from build123d import *

# Parameters (mm, degrees)
SKETCH1_W                      = 86
SKETCH1_H                      = 16
BOSS_EXTRUDE1_DEPTH            = 3
M3_CLEARANCE_HOLE1_D           = 3.4
M3_CLEARANCE_HOLE1_CSINK_D     = 3.45
M3_CLEARANCE_HOLE1_CSINK_ANGLE = 90


with BuildPart() as part:
    # Sketch1 → Boss-Extrude1 (new body)
    with BuildSketch(Plane.XY):
        with Locations((43, 8)):
            Rectangle(SKETCH1_W, SKETCH1_H)
    extrude(amount=BOSS_EXTRUDE1_DEPTH)

    # M3 Clearance Hole1 (through all)
    with Locations(Plane.XY.offset(3)):
        with Locations((5.115834522, 13), (5.115834522, 3), (79.115834522, 13), (79.115834522, 3)):
            CounterSinkHole(M3_CLEARANCE_HOLE1_D / 2, M3_CLEARANCE_HOLE1_CSINK_D / 2, counter_sink_angle=M3_CLEARANCE_HOLE1_CSINK_ANGLE)


solid = part.part
Check sheet for the modelled part. Datum: model origin and axes. Units: mm. Coordinates: 2 decimals unless noted, no trailing zeros. Write each loop counter-clockwise with the first axis right and the second up, starting at its lowest first coordinate (ties: lowest second). Pieces come first, ordered by that corner, then holes.
Item 1: Depth check by flat-ended pin: pin 1 Ø2 at (x, y) = (5.12, 3) entering from +Z. Enter the tip coordinate at first touch or a pass-through.
Numbers:
pin 1: passes through
Item 2: Cross-section at A-A on z = 0.75. Record the boundary of the cut face in (x, y), then the cut area to 3 significant figures.
Numbers:
outline: (0, 0) - (86, 0) - (86, 16) - (0, 16) - close; hole circle Ø3.4 at (5.12, 3); hole circle Ø3.4 at (5.12, 13); hole circle Ø3.4 at (79.12, 3); hole circle Ø3.4 at (79.12, 13)
area: 1,340 mm2
Item 3: Mould release check, pull along X, two halves, no side actions. Record for faces 1 (the face through (86, 8, 1)), 2 (the face through (4.2, 4.43, 1.47)), 3 (the face through (42, 8, 0)): released by +X, released by -X, zero draft, split by the parting line, or undercut.
Numbers:
face 1: released by +X
face 2: undercut
face 3: zero draft
Item 4: Cross-section at C-C on x = 5. Count the separate pieces of the cut face and the enclosed holes in it, then the cut area to 3 significant figures.
Numbers:
separate pieces: 3
enclosed holes: 0
area: 27.6 mm2
Item 5: Cross-section at B-B on y = 3. Record the boundary of the cut face in (x, z) (3 decimals).
Numbers:
outline: (0, 0) - (3.416, 0) - (3.416, 2.975) - (3.391, 3) - (0, 3) - close; (6.816, 0) - (77.416, 0) - (77.416, 2.975) - (77.391, 3) - (6.841, 3) - (6.816, 2.975) - close; (80.816, 0) - (86, 0) - (86, 3) - (80.841, 3) - (80.816, 2.975) - close
Item 6: Scan lines: probe 1 along X at (y, z) = (3, 0.8); probe 2 along X at (y, z) = (14, 1.15). Record each from-to range of solid material in increasing order.
Numbers:
probe 1: x = 0 to 3.42, 6.82 to 77.42, 80.82 to 86
probe 2: x = 0 to 3.74, 6.49 to 77.74, 80.49 to 86
